Verification items for the finished model (mm, model axes). A direction names the side the tool comes from. Coordinates: 2 decimals unless noted, no trailing zeros. Loops run counter-clockwise (first coordinate to the right, second up) from the corner with the lowest first, then second, coordinate; pieces in that order, holes last. Notation, with made-up numbers: (62.5, 1) - (101.5, 1) arc R32 ccw to (101.5, 29) - close; hole circle Ø2 at (-35.75, 57). An arc over 180 degrees is marked (long way). One line per item, written item: value. Start each with the question number.
(1) Section check D-D (z = -18). Record the boundary of the cut face in (x, y), plus the area to 3 significant figures.
(2) Section check B-B (x = 36.75). Record the boundary of the cut face in (y, z).
(3) Thickness scan on probe 1 along Y at (x, z) = (5.75, -7); probe 2 along X at (y, z) = (-36.75, -5.5); probe 3 along Y at (x, z) = (36, -7). Record the ranges inside material, lowest first. Write a range as [from, to].
(4) Section check A-A (z = -2). Record the boundary of the cut face in (x, y), plus the area to 3 significant figures.
(5) Draft check along X on faces 1 (the face through (40.5, -2, -19.8)), 2 (the face through (6.075, -35.286, -5.057)), 3 (the face through (23.748, -21.14, 10.381)). Enter one of: +X half, -X half, draft (parallel to the pull), parting line (faces both ways), or undercut.
(6) Set-up check for faces 4 (the face through (40, -41, -20)), 5 (the face through (6, -6, -10)): record each of +Z, -Z, +X, -X, +Y, -Y from which the full face is reachable in a straight line by a thin tool's end or side.
(7) Section check C-C (y = -5.75). Record the boundary of the cut face in (x, z).
(8) Gauge pin test, flat ends, axial feed: P1, Ø0.9, axis at x = 6, y = -5.5, coming from the +Z side; P2, Ø4, axis at x = 13, y = -15, coming from the +Z side; P3, Ø3.5, axis at x = 5.5, y = -37, coming from the +Z side. Record the tip position at first contact, or that the pin passes through.
Autodesk Fusion 360 part; units mm, degrees
sketch "Sketch1" plane through (0, 0, 0) normal (0, 0, 1) x (1, 0, 0)
  line L0 (0, 0) -> (42.5, 0)
  line L1 (42.5, 0) -> (42.5, -42.5)
  line L2 (42.5, -42.5) -> (0, -42.5)
  line L3 (0, -42.5) -> (0, 0)
  dimension "d1" = 42.5
  dimension "d2" = 42.5
extrude "Extrude1" add sketch "Sketch1" against normal blind 39
sketch "Sketch2" plane through (0, 0, 0) normal (0, 0, 1) x (-1, 0, 0)
  line L0 (0, 42.5) -> (-42.5, 42.5)
  line L1 (-42.5, 42.5) -> (-42.5, 0)
  line L2 (-42.5, 0) -> (0, 0)
  line L3 (0, 0) -> (0, 42.5)
  line L4 (0, 0) -> (-42.5, 42.5)
  line L5 (-42.5, 0) -> (0, 42.5)
  line L6 (-5.75, 5.75) -> (-36.75, 5.75)
  line L7 (-36.75, 5.75) -> (-36.75, 36.75)
  line L8 (-36.75, 36.75) -> (-5.75, 36.75)
  line L9 (-5.75, 36.75) -> (-5.75, 5.75)
  circle A0 centre (-5.75, 5.75) radius 1.5
  circle A1 centre (-36.75, 5.75) radius 1.5
  circle A2 centre (-5.75, 36.75) radius 1.5
  circle A3 centre (-36.75, 36.75) radius 1.5
  dimension "d5" = 31
  dimension "d6" = 3
  dimension "d7" = 3
  dimension "d8" = 3
  dimension "d9" = 3
extrude "Extrude2" cut sketch "Sketch2" against normal blind 10 contours L5 L9 A2 | L5 L8 A2 | L4 L8 A3 | L4 L7 A3 | L4 L6 A0 | L4 L9 A0 | L5 L9 A2 | L5 L8 A2 | L5 L7 A1 | L5 L6 A1 | L4 L8 A3 | L4 L7 A3 | L4 L6 A0 | L4 L9 A0 | L5 L7 A1 | L5 L6 A1
chamfer "Chamfer1" distance 0.25 angle 45 4 edges at (7.1485, -6.2924, 0) (38.1485, -6.2924, 0) (38.1485, -37.2924, 0) (7.1485, -37.2924, 0)
thread "Thread1"
chamfer "Chamfer2" distance 4 angle 45 4 edges at (42.5, 0, -19.5) (0, 0, -19.5) (0, -42.5, -19.5) (42.5, -42.5, -19.5)
sketch "Sketch3" plane through (0, 0, 0) normal (0, 0, 1) x (-1, 0, 0)
  circle A0 centre (-36.75, 36.75) radius 1.75
  circle A1 centre (-5.75, 5.75) radius 1.75
  line L0 (-38.5, 42.5) -> (-42.5, 38.5)
  line L1 (-42.5, 38.5) -> (-42.5, 4)
  line L2 (-42.5, 4) -> (-38.5, 0)
  line L3 (-38.5, 0) -> (-4, 0)
  line L4 (-4, 0) -> (0, 4)
  line L5 (0, 4) -> (0, 38.5)
  line L6 (0, 38.5) -> (-4, 42.5)
  line L7 (-4, 42.5) -> (-38.5, 42.5)
  circle A2 centre (-36.75, 5.75) radius 1.75
  circle A3 centre (-5.75, 36.75) radius 1.75
  line L8 (-5.75, 5.75) -> (-36.75, 36.75)
  line L9 (-36.75, 36.75) -> (-36.75, 5.75)
  line L10 (-36.75, 5.75) -> (-5.75, 36.75)
  circle A4 centre (-21.25, 21.25) radius 11
  dimension "d14" = 22
extrude "Extrude3" add sketch "Sketch3" along normal blind 2 contours L8 L10 A4 | L8 L10 A4 | L8 L10 A4 | L8 L10 A4
sketch "Sketch4" plane through (0, 0, 2) normal (0, 0, 1) x (-1, 0, 0)
  circle A0 centre (-21.25, 21.25) radius 11
  circle A1 centre (-21.25, 21.25) radius 2.5
  dimension "d17" = 5
extrude "Extrude4" add sketch "Sketch4" along normal blind 17 contours A1
Responses:
1. outline: (0, -38.5) - (4, -42.5) - (38.5, -42.5) - (42.5, -38.5) - (42.5, -4) - (38.5, 0) - (4, 0) - (0, -4) - close
1. area: 1,770 mm²
2. outline: (-42.5, -39) - (0, -39) - (0, 0) - (-4, 0) - (-4.25, -0.25) - (-4.25, -10) - (-7.25, -10) - (-7.25, -0.25) - (-7.5, 0) - (-35, 0) - (-35.25, -0.25) - (-35.25, -10) - (-38.25, -10) - (-38.25, -0.25) - (-38.5, 0) - (-42.5, 0) - close
3. probe 1: y = [-42.5, -38.25], [-35.25, -7.25], [-4.25, 0]
3. probe 2: x = [0, 4.25], [7.25, 35.25], [38.25, 42.5]
3. probe 3: y = [-42.5, -38.05], [-35.45, -7.05], [-4.45, 0]
4. outline: (0, -38.5) - (4, -42.5) - (38.5, -42.5) - (42.5, -38.5) - (42.5, -4) - (38.5, 0) - (4, 0) - (0, -4) - close; hole circle Ø3 at (5.75, -36.75); hole circle Ø3 at (5.75, -5.75); hole circle Ø3 at (36.75, -36.75); hole circle Ø3 at (36.75, -5.75)
4. area: 1,750 mm²
5. face 1: +X half
5. face 2: undercut
5. face 3: parting line
6. face 4: +Z, -Z, +X, -Y
6. face 5: +Z
7. outline: (0, -39) - (42.5, -39) - (42.5, 0) - (38.5, 0) - (38.25, -0.25) - (38.25, -10) - (35.25, -10) - (35.25, -0.25) - (35, 0) - (7.5, 0) - (7.25, -0.25) - (7.25, -10) - (4.25, -10) - (4.25, -0.25) - (4, 0) - (0, 0) - close
8. P1: stops at z = -10
8. P2: stops at z = 2
8. P3: stops at z = 0
